Study the drawing (mm; zero at the part's minimum x, y, z) and answer. A direction names the side the tool comes from. Round coordinates to 2 decimals unless told otherwise and drop trailing zeros. Loops run counter-clockwise (first coordinate to the right, second up) from the corner with the lowest first, then second, coordinate; pieces in that order, holes last. Notation, with made-up numbers: (-39, 9.5) -> (19, 9.5) arc R26 cw to (19, 38.5) -> close; hole circle Ø8 at (76.5, 87). An arc over 180 degrees is marked (long way). Write each question's results on one line, items separated by ' | '. Start each with the question number.
(1) Straight lines are drawn through the part: probe 1 along Y at (x, z) = (12.5, 55.5); probe 2 along Y at (x, z) = (2.5, 22.5). For each, find the intervals that lie inside material, in ascending order.
(2) A flat-ended cylindrical pin translates along its axis: pin 1 (3 mm diameter, centred on x = 19, z = 56.5, fed in from -Y). Find the tip coordinate at first contact, or state that the pin passes through.
(3) The part is cut by section A-A (y = 16.5). Determine the outline of the cut face in (x, z), plus the area to 3 significant figures.
(4) The part is cut by section B-B (z = 54). Determine the outline of the cut face in (x, y).
(5) Determine the mould class of the marked faces 3, 4 and 5 for opening direction Y: released by +Y, released by -Y, zero draft, split by the parting line, or undercut.
(6) For the marked faces 1 and 2, determine the directions among +Z, -Z, +X, -X, +Y, -Y from which every point of the face is accessible in a straight line to the end or side of a thin tool.
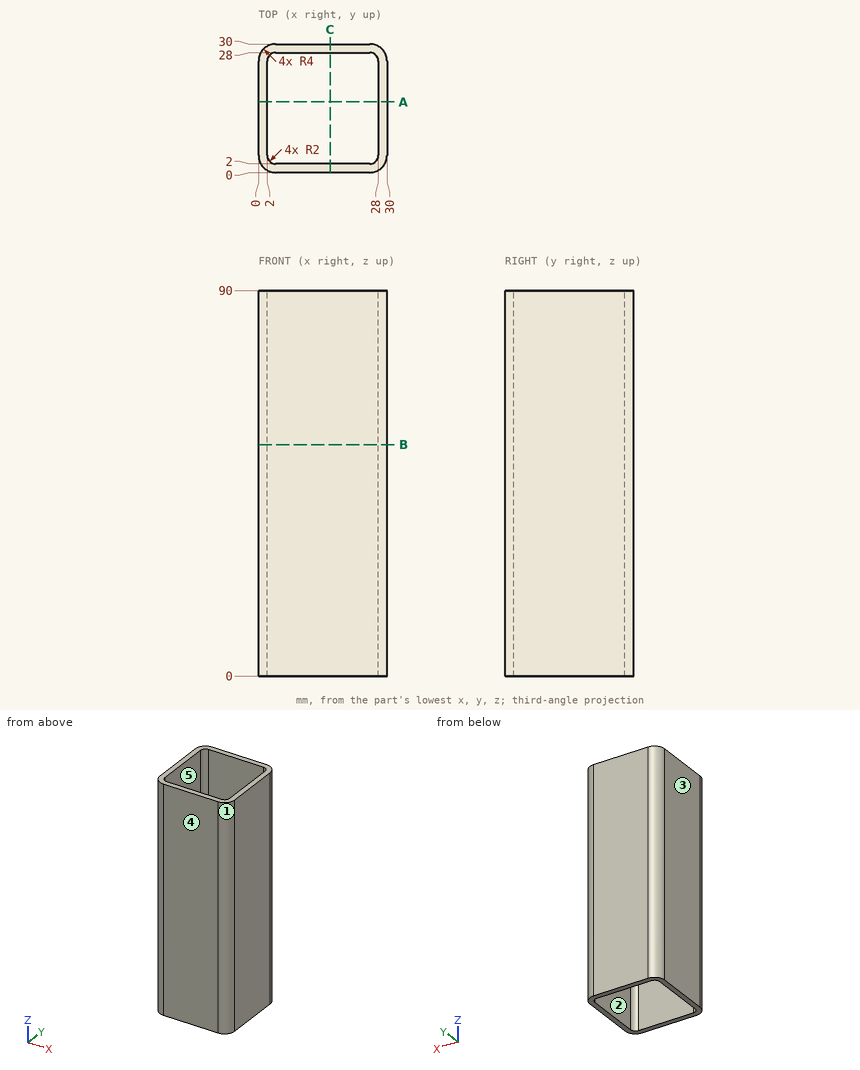
Checked values:
1) probe 1: y = 0 to 2, 28 to 30 | probe 2: y = 0.29 to 2.68, 27.32 to 29.71
2) pin 1: stops at y = 0
3) outline: (0, 0) -> (2, 0) -> (2, 90) -> (0, 90) -> close; (28, 0) -> (30, 0) -> (30, 90) -> (28, 90) -> close | area: 360 mm2
4) outline: (0, 4) arc R4 ccw to (4, 0) -> (26, 0) arc R4 ccw to (30, 4) -> (30, 26) arc R4 ccw to (26, 30) -> (4, 30) arc R4 ccw to (0, 26) -> close; hole (2, 4) arc R2 ccw to (4, 2) -> (26, 2) arc R2 ccw to (28, 4) -> (28, 26) arc R2 ccw to (26, 28) -> (4, 28) arc R2 ccw to (2, 26) -> close
5) face 3: zero draft | face 4: released by -Y | face 5: undercut
6) face 1: +Z, -Z, +X, -Y | face 2: +Z, -Z
